Geometry: see drawing. Coordinates: mm, zero at the bounding-box minimum. A direction names the side the tool comes from. Give positions to 0.01 mm unless a question says otherwise; leave off trailing zeros. Order: outer loops, then holes, each group sorted by start corner. A loop starts at its lowest first (then second) coordinate and runs counter-clockwise, first axis right, second up. Notation, with made-up numbers: M -37.75,-8.5 L 5.25,-8.5 A16 ccw 5.25,3.5 Z; hole C 73.25,-31 d8. An arc over 180 degrees is marked long. Return JSON: item names as keys, results as strings.
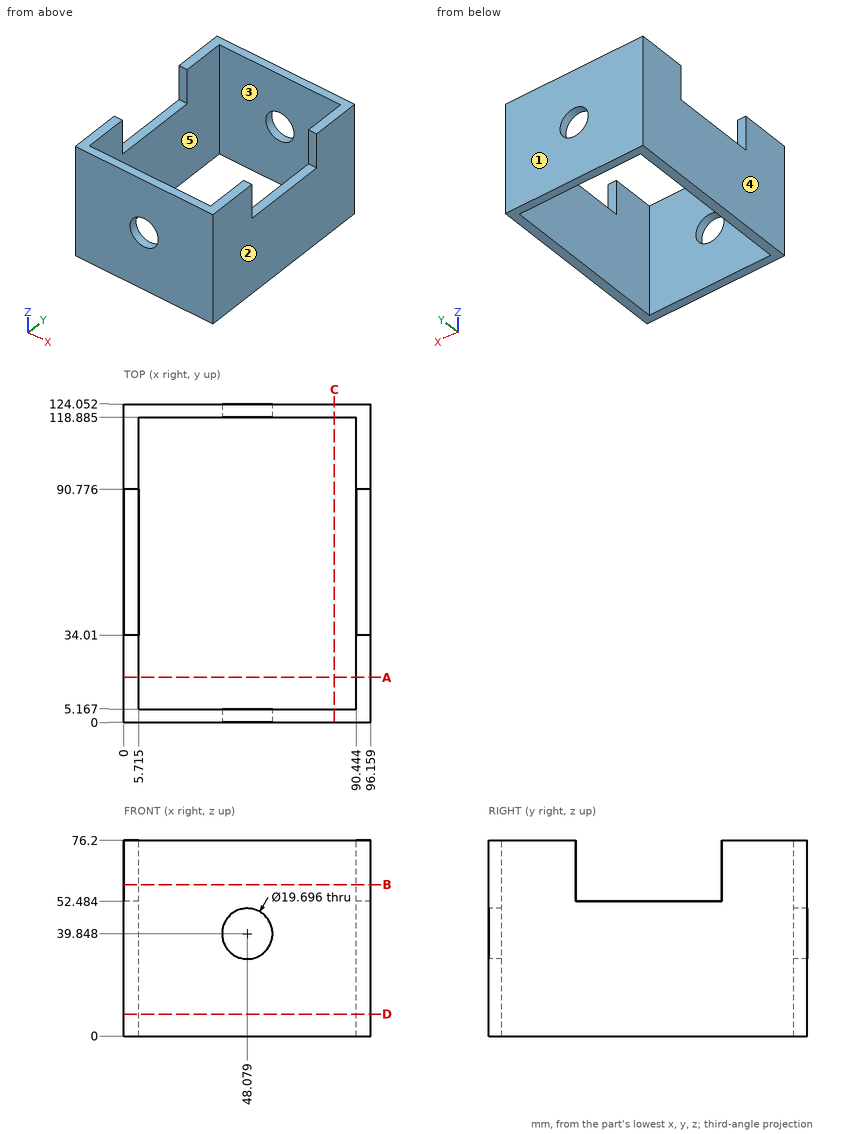
1. Ray query, probe 1 along X at (y, z) = (92, 59.5) (1 decimal); probe 2 along Y at (x, z) = (72, 32) (1 decimal). Return the intervals inside material, ascending.
Evaluation:
{"probe 1": "x = 0 to 5.7, 90.4 to 96.2", "probe 2": "y = 0 to 5.2, 118.9 to 124.1"}
2. Section query D-D (z = 8.5). Return loops of the section in (x, y) (1 decimal), then the cut area to 3 significant figures.
Evaluation:
{"outline": "M 0,0 L 96.2,0 L 96.2,124.1 L 0,124.1 Z; hole M 5.7,5.2 L 90.4,5.2 L 90.4,118.9 L 5.7,118.9 Z", "area": "2,290 mm^2"}
3. First-contact query: pin 1 (4.5 mm diameter, centred on x = 94, y = 63, fed in from +Z); pin 2 (16 mm diameter, centred on x = 48.08, z = 39.85, fed in from +Y). Flat tips, straight axial feed; report the tip coordinate or a pass-through.
Evaluation:
{"pin 1": "stops at z = 52.48", "pin 2": "passes through"}
4. Draft query along X for the marked faces 1, 2 and 3. Return one class per face: pulls with the +X half, pulls with the -X half, needs draft (parallel to the pull), parting line crosses it, or undercut.
Evaluation:
{"face 1": "needs draft", "face 2": "pulls with the +X half", "face 3": "undercut"}
5. Section query B-B (z = 59). Return loops of the section in (x, y) (1 decimal).
Evaluation:
{"outline": "M 0,0 L 96.2,0 L 96.2,34 L 90.4,34 L 90.4,5.2 L 5.7,5.2 L 5.7,34 L 0,34 Z; M 0,90.8 L 5.7,90.8 L 5.7,118.9 L 90.4,118.9 L 90.4,90.8 L 96.2,90.8 L 96.2,124.1 L 0,124.1 Z"}
6. Set-up query: the marked faces 4 and 5. Return all of +Z, -Z, +X, -X, +Y, -Y with unobstructed straight access to the full face (end or side cutting, diameter ignored); none if empty.
Evaluation:
{"face 4": "+Z, -Z, -X, +Y, -Y", "face 5": "+Z, -Z"}
7. Section query C-C (x = 82). Return loops of the section in (y, z) (1 decimal).
Evaluation:
{"outline": "M 0,0 L 5.2,0 L 5.2,76.2 L 0,76.2 Z; M 118.9,0 L 124.1,0 L 124.1,76.2 L 118.9,76.2 Z"}
8. Section query A-A (y = 17.5). Return loops of the section in (x, z) (1 decimal), then the cut area to 3 significant figures.
Evaluation:
{"outline": "M 0,0 L 5.7,0 L 5.7,76.2 L 0,76.2 Z; M 90.4,0 L 96.2,0 L 96.2,76.2 L 90.4,76.2 Z", "area": "871 mm^2"}
